Geometry: final body of the model. Coordinates: model frame, mm. A direction names the side the tool comes from. Round coordinates to 2 decimals unless told otherwise and drop trailing zeros. Write each loop counter-clockwise with the first axis right and the second up, starting at its lowest first coordinate (ties: lowest second). Pieces come first, ordered by that corner, then holes. Notation, with made-up numbers: (55, 4) - (114, 4) arc R18 cw to (114, 39) - close; hole circle Ø3 at (6.5, -33.75). An arc over 180 degrees is marked (long way). Use a Markdown table: item, result. Add a question column.
```python
from build123d import *

# Parameters (mm, degrees)
F0_W     = 72
F0_H     = 37.2
F0_W_2   = 7.75
F0_H_2   = 6
F0_W_3   = 8.5
F0_W_4   = 67
F0_H_3   = 9
F0_H_4   = 7.35
F0_W_5   = 14
F1_DEPTH = 1
F0_W_6   = 1
F2_DEPTH = 25
F3_DEPTH = 50
F5_R     = 1.45
F6_DEPTH = 1
F7_SIZE  = 0.5
F8_R     = 1.5


with BuildPart() as f1:
    # F0 (on Top) → F1 (new body)
    with BuildSketch(Plane.XY):
        Rectangle(F0_W, F0_H)
        with Locations((-29.625, -14.6)):
            Rectangle(F0_W_2, F0_H_2, mode=Mode.SUBTRACT)
        with Locations((-20, -14.6)):
            Rectangle(F0_W_3, F0_H_2, mode=Mode.SUBTRACT)
        with Locations((-10, -14.6)):
            Rectangle(F0_W_3, F0_H_2, mode=Mode.SUBTRACT)
        with Locations((0, -14.6)):
            Rectangle(F0_W_3, F0_H_2, mode=Mode.SUBTRACT)
        with Locations((10, -14.6)):
            Rectangle(F0_W_3, F0_H_2, mode=Mode.SUBTRACT)
        with Locations((20, -14.6)):
            Rectangle(F0_W_3, F0_H_2, mode=Mode.SUBTRACT)
        with Locations((29.625, -14.6)):
            Rectangle(F0_W_2, F0_H_2, mode=Mode.SUBTRACT)
        with Locations((0, -5.1)):
            Rectangle(F0_W_4, F0_H_3, mode=Mode.SUBTRACT)
        with Locations((-29.625, 5.075)):
            Rectangle(F0_W_2, F0_H_4, mode=Mode.SUBTRACT)
        with Locations((-20, 5.075)):
            Rectangle(F0_W_3, F0_H_4, mode=Mode.SUBTRACT)
        with Locations((-10, 5.075)):
            Rectangle(F0_W_3, F0_H_4, mode=Mode.SUBTRACT)
        with Locations((-29.625, 13.925)):
            Rectangle(F0_W_2, F0_H_4, mode=Mode.SUBTRACT)
        with Locations((-20, 13.925)):
            Rectangle(F0_W_3, F0_H_4, mode=Mode.SUBTRACT)
        with Locations((-10, 13.925)):
            Rectangle(F0_W_3, F0_H_4, mode=Mode.SUBTRACT)
        with Locations((0, 5.075)):
            Rectangle(F0_W_3, F0_H_4, mode=Mode.SUBTRACT)
        with Locations((10, 5.075)):
            Rectangle(F0_W_3, F0_H_4, mode=Mode.SUBTRACT)
        with Locations((0, 13.925)):
            Rectangle(F0_W_3, F0_H_4, mode=Mode.SUBTRACT)
        with Locations((10, 13.925)):
            Rectangle(F0_W_3, F0_H_4, mode=Mode.SUBTRACT)
        with Locations((25.25, 11.1)):
            Rectangle(F0_W_5, F0_H_3, mode=Mode.SUBTRACT)
    extrude(amount=F1_DEPTH)

    # F0 (on Top) → F2 (join)
    with BuildSketch(Plane.XY):
        Polygon((36, 18.6), (37, 18.6), (37, 19.6), (-37, 19.6), (-37, 18.6), (-36, 18.6), align=None)
        Polygon((37, -19.6), (37, -18.6), (36, -18.6), (-36, -18.6), (-37, -18.6), (-37, -19.6), align=None)
        with Locations((-36.5, 0)):
            Rectangle(F0_W_6, F0_H)
        with Locations((36.5, 0)):
            Rectangle(F0_W_6, F0_H)
    extrude(amount=F2_DEPTH)

    # F0 (on Top) → F3 (join)
    with BuildSketch(Plane.XY):
        Polygon((38.5, -19.6), (37, -19.6), (-37, -19.6), (-38.5, -19.6), (-38.5, -21.1), (38.5, -21.1), align=None)
        Polygon((-37, 18.6), (-37, 19.6), (-38.5, 19.6), (-38.5, -19.6), (-37, -19.6), (-37, -18.6), align=None)
        Polygon((37, 19.6), (37, 18.6), (37, -18.6), (37, -19.6), (38.5, -19.6), (38.5, 19.6), align=None)
        Polygon((-37, 19.6), (37, 19.6), (38.5, 19.6), (38.5, 21.1), (-38.5, 21.1), (-38.5, 19.6), align=None)
    extrude(amount=F3_DEPTH)

    # F5 (on face) → F6 (join)
    with BuildSketch(Plane.YZ.offset(-37)):
        with Locations((3.15, 30.17)):
            Circle(F5_R)
    extrude(amount=F6_DEPTH)

    # F7
    f7_edges = [f1.edges().sort_by_distance(p)[0] for p in [
        (-36, 1.7, 30.17),
    ]]
    chamfer(f7_edges, length=F7_SIZE)

    # F8
    f8_edges = [f1.edges().sort_by_distance(p)[0] for p in [
        (-36, 2.2, 30.17),
    ]]
    fillet(f8_edges, radius=F8_R)


solid = f1.part
```
1) Draft query along Y for faces 1 (the flat face through (-1, 0, 0)), 2 (the flat face through (-1, 18.6, 13)), 3 (the flat face through (36, 0, 13)), 4 (the flat face through (1, 21.1, 25)). Return one class per face: released by +Y, released by -Y, zero draft, split by the parting line, or undercut.
2) Section C-C, the plane y = 7.5. State how many separate pieces and enclosed holes the cut face has, then the cut area to 3 significant figures.
3) Pin query (flat end, axial travel): P1, Ø10, axis at x = 16, y = 2.5, coming from the +Z side. Return the tip coordinate at first contact, or that it passes through.
4) Set-up query: faces 5 (the flat face through (1, -19.6, 37)), 6 (the cylindrical face through (-36.754, 2.961, 31.608)), 7 (the flat face through (-38.5, 0, 25)). Return all of +Z, -Z, +X, -X, +Y, -Y with unobstructed straight access to the full face (end or side cutting, diameter ignored); none if empty.
5) Section A-A, the plane x = -2. Return the cut outline in (y, z), then the cut area to 4 significant figures.
6) Material intervals for L1, parallel to X at y = 18, z = 12.5; L2, parallel to X at y = -0.5, z = 37; L3, parallel to Y at x = 4, z = 27, sorted ascending. Write a range as from..to.
7) Section B-B, the plane z = 17.5. Return the cut outline in (x, y).
Output values:
| question | item | result |
|---|---|---|
| 1 | face 1 | zero draft |
| 1 | face 2 | undercut |
| 1 | face 3 | undercut |
| 1 | face 4 | released by +Y |
| 2 | separate pieces | 7 |
| 2 | enclosed holes | 0 |
| 2 | area | 216 mm^2 |
| 3 | P1 | stops at z = 1 |
| 4 | face 5 | +Z |
| 4 | face 6 | none |
| 4 | face 7 | +Z, -Z, -X, +Y, -Y |
| 5 | outline | (-21.1, 0) - (-17.6, 0) - (-17.6, 1) - (-18.6, 1) - (-18.6, 25) - (-19.6, 25) - (-19.6, 50) - (-21.1, 50) - close; (-11.6, 0) - (-9.6, 0) - (-9.6, 1) - (-11.6, 1) - close; (-0.6, 0) - (1.4, 0) - (1.4, 1) - (-0.6, 1) - close; (8.75, 0) - (10.25, 0) - (10.25, 1) - (8.75, 1) - close; (17.6, 0) - (21.1, 0) - (21.1, 50) - (19.6, 50) - (19.6, 25) - (18.6, 25) - (18.6, 1) - (17.6, 1) - close |
| 5 | area | 207.5 mm^2 |
| 6 | L1 | x = -38.5..-36, 36..38.5 |
| 6 | L2 | x = -38.5..-37, 37..38.5 |
| 6 | L3 | y = -21.1..-19.6, 19.6..21.1 |
| 7 | outline | (-38.5, -21.1) - (38.5, -21.1) - (38.5, 21.1) - (-38.5, 21.1) - close; hole (-36, -18.6) - (36, -18.6) - (36, 18.6) - (-36, 18.6) - close |
